```python
from build123d import *

# Parameters (mm, degrees)
SKETCH_1_W             = 50
SKETCH_1_H             = 12
EXTRUDE_1_DEPTH        = 50
HOLE_WIZARD_M4_1_D     = 3.3
HOLE_WIZARD_M4_1_DEPTH = 10.1
HOLE_WIZARD_M4_1_TIP   = 0.991420021
SKETCH_5_R             = 10
SKETCH_5_R_2           = 1.6
CUT_EXTRUDE_1_DEPTH    = 50


with BuildPart() as part:
    # 草图1 → 凸台-拉伸1 (new body)
    with BuildSketch(Plane.XY):
        with Locations((-1.474142426, -7.925704975)):
            Rectangle(SKETCH_1_W, SKETCH_1_H)
    extrude(amount=EXTRUDE_1_DEPTH)

    # M4 螺纹孔1
    with Locations(Plane(origin=(0, 0, 0), x_dir=(-1, 0, 0), z_dir=(0, 0, -1))):
        with Locations((-4.525857574, -7.925704975), (14.474142426, -7.925704975)):
            Hole(HOLE_WIZARD_M4_1_D / 2, depth=HOLE_WIZARD_M4_1_DEPTH)
            with Locations((0, 0, -(HOLE_WIZARD_M4_1_DEPTH + HOLE_WIZARD_M4_1_TIP / 2))):  # 118° drill point
                Cone(0, HOLE_WIZARD_M4_1_D / 2, HOLE_WIZARD_M4_1_TIP, mode=Mode.SUBTRACT)

    # 草图5 → 切除-拉伸1 (cut)
    with BuildSketch(Plane(origin=(0, -1.925704975, 0), x_dir=(1, 0, 0), z_dir=(0, 1, 0))):
        with Locations((4.525857574, -25.389445239)):
            Circle(SKETCH_5_R)
        with Locations((12.025857574, -12.399064182)):
            Circle(SKETCH_5_R_2)
        with Locations((12.025857574, -38.379826296)):
            Circle(SKETCH_5_R_2)
        with Locations((-10.474142426, -25.389445239)):
            Circle(SKETCH_5_R_2)
    extrude(amount=-CUT_EXTRUDE_1_DEPTH, mode=Mode.SUBTRACT)


solid = part.part
```
Read the model definition and answer for the solid it produces. Units are mm, in the model's axes. A direction names the side the tool comes from. Round coordinates to 2 decimals unless told otherwise and drop trailing zeros. Write each loop counter-clockwise with the first axis right and the second up, starting at its lowest first coordinate (ties: lowest second). Pieces come first, ordered by that corner, then holes. Notation, with made-up numbers: (39, -38) - (98, -38) arc R24 ccw to (98, -9) - close; hole circle Ø4 at (-30.5, 30.5). An arc over 180 degrees is marked (long way). One line per item, written item: value.
Q1. Find section A-A (x = 0). Determine the outline of the cut face in (y, z), and give its area (3 significant figures).
The answers:
outline: (-13.93, 0) - (-1.93, 0) - (-1.93, 16.47) - (-13.93, 16.47) - close; (-13.93, 34.31) - (-1.93, 34.31) - (-1.93, 50) - (-13.93, 50) - close
area: 386 mm2
Q2. For a pull along Y with two mould halves and no side action, classify faces 3 (the cylindrical face through (-14.832, -9.536, 5.121)), 4 (the flat face through (-2, -8, 0)), 5 (the flat face through (-7, -13.926, 25)) as pulls with the +Y half, pulls with the -Y half, needs draft (parallel to the pull), parting line crosses it, or undercut.
The answers:
face 3: undercut
face 4: needs draft
face 5: pulls with the -Y half
Q3. Find section D-D (z = 9.5). Determine the outline of the cut face in (x, y), and give its area (3 significant figures).
The answers:
outline: (-26.47, -13.93) - (23.53, -13.93) - (23.53, -1.93) - (-26.47, -1.93) - close; hole circle Ø3.3 at (-14.47, -7.93); hole circle Ø3.3 at (4.53, -7.93)
area: 583 mm2
Q4. Straight lines are drawn through the part: line 1 (Z direction, x = -10.5, y = -6.5); line 2 (Z direction, x = 13, y = -7); line 3 (X direction, y = -8.25, z = 29). For each, find the intervals that lie inside material, in ascending order. Write a range as from..to.
The answers:
line 1: z = 0..23.79, 26.99..50
line 2: z = 0..11.13, 13.67..20.08, 30.7..37.11, 39.65..50
line 3: x = -26.47..-4.8, 13.85..23.53
Q5. Which of the six approach directions +Z, -Z, +X, -X, +Y, -Y give full straight-line access (tool end or side, diameter ignored) to faces 1 (the flat face through (23.526, -8, 25)), 2 (the cylindrical face through (6.05, -8.56, 5.12))?
The answers:
face 1: +Z, -Z, +X, +Y, -Y
face 2: -Z
Q6. Find section C-C (y = -13). Determine the outline of the cut face in (x, z), and give its area (3 significant figures).
The answers:
outline: (-26.47, 0) - (23.53, 0) - (23.53, 50) - (-26.47, 50) - close; hole circle Ø3.2 at (-10.47, 25.39); hole circle Ø20 at (4.53, 25.39); hole circle Ø3.2 at (12.03, 12.4); hole circle Ø3.2 at (12.03, 38.38)
area: 2,160 mm2
Q7. Find section B-B (z = 30). Determine the outline of the cut face in (x, y).
The answers:
outline: (-26.47, -13.93) - (-4.35, -13.93) - (-4.35, -1.93) - (-26.47, -1.93) - close; (13.4, -13.93) - (23.53, -13.93) - (23.53, -1.93) - (13.4, -1.93) - close
